Can you work these out from the drawing? Everything is in mm from the part's minimum corner. A direction names the side the tool comes from. Round coordinates to 2 decimals unless told otherwise and drop trailing zeros. Loops run counter-clockwise (first coordinate to the right, second up) from the corner with the lowest first, then second, coordinate; pieces in that order, holes last. Notation, with made-up numbers: (38, 65) -> (62, 65) arc R29 ccw to (62, 89) -> close; hole circle Ø7 at (45, 88.25). An arc over 180 degrees is marked (long way). One line per item, written item: value.
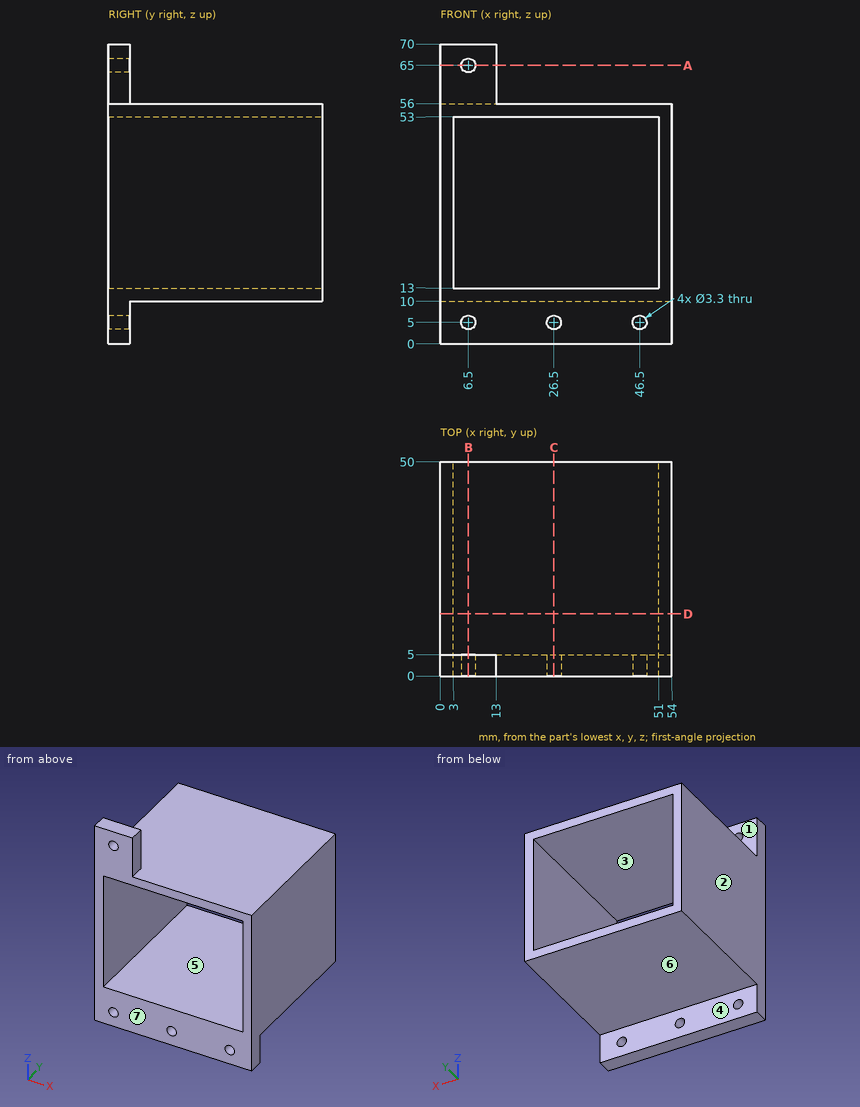
(1) Please list where these lines run through material, in increasing order: L1, parallel to X at y = 1.1, z = 5; L2, parallel to X at y = 31, z = 29; L3, parallel to Z at x = 42.5, y = 43.
Results below:
L1: x = 0 to 4.85, 8.15 to 24.85, 28.15 to 44.85, 48.15 to 54
L2: x = 0 to 3, 51 to 54
L3: z = 10 to 13, 53 to 56
(2) On a 3-axis mill with a long thin cutter (end or side, diameter ignored), from which of +Z, -Z, +X, -X, +Y, -Y can I reach the whole of each face in a straight line? I mean the marked faces 1, 2, 3 and 4. Say none if no direction works.
Results below:
face 1: +Z, +X, -X, +Y
face 2: +Z, -Z, -X, +Y, -Y
face 3: +Y, -Y
face 4: -Z, +X, -X, +Y
(3) Imagine slicing it at C-C on x = 26.5. Write out the boundary of the cut face in (y, z), then the cut area to 4 significant figures.
Results below:
outline: (0, 0) -> (5, 0) -> (5, 3.35) -> (0, 3.35) -> close; (0, 6.65) -> (5, 6.65) -> (5, 10) -> (50, 10) -> (50, 13) -> (0, 13) -> close; (0, 53) -> (50, 53) -> (50, 56) -> (0, 56) -> close
area: 333.5 mm²
(4) Imagine slicing it at B-B on x = 6.5. Write out the boundary of the cut face in (y, z), then the cut area to 3 significant figures.
Results below:
outline: (0, 0) -> (5, 0) -> (5, 3.35) -> (0, 3.35) -> close; (0, 6.65) -> (5, 6.65) -> (5, 10) -> (50, 10) -> (50, 13) -> (0, 13) -> close; (0, 53) -> (50, 53) -> (50, 56) -> (5, 56) -> (5, 63.35) -> (0, 63.35) -> close; (0, 66.65) -> (5, 66.65) -> (5, 70) -> (0, 70) -> close
area: 387 mm²
(5) We'd pull the mould along Z, two halves only. Please class the marked faces 5, 6 and 7: +Z half, -Z half, draft (parallel to the pull), parting line (faces both ways), or undercut.
Results below:
face 5: undercut
face 6: -Z half
face 7: draft
(6) Imagine slicing it at D-D on y = 14.5. Write out the boundary of the cut face in (x, z), then the cut area to 3 significant figures.
Results below:
outline: (0, 10) -> (54, 10) -> (54, 56) -> (0, 56) -> close; hole (3, 13) -> (51, 13) -> (51, 53) -> (3, 53) -> close
area: 564 mm²
(7) For pin 1 Ø15 at (x, y) = (28, 23) entering from +Z; pin 2 Ø4 at (x, y) = (47.5, 8) entering from -Z; pin 3 Ø5 at (x, z) = (17.5, 6) entering from +Y, each with a flat end and sliding along its axis, tell me the tip position at first contact or that it passes through.
Results below:
pin 1: stops at z = 56
pin 2: stops at z = 10
pin 3: stops at y = 5
(8) Imagine slicing it at A-A on z = 65. Write out the boundary of the cut face in (x, y), then the cut area to 3 significant figures.
Results below:
outline: (0, 0) -> (4.85, 0) -> (4.85, 5) -> (0, 5) -> close; (8.15, 0) -> (13, 0) -> (13, 5) -> (8.15, 5) -> close
area: 48.5 mm²
